Geometry check sheet. Reference: the model listing, model coordinates, mm. Face numbers are marked on the shaded views. A direction names the side the tool comes from. Give positions to 0.01 mm unless a question says otherwise; leave off trailing zeros. Loops run counter-clockwise (first coordinate to the right, second up) from the corner with the lowest first, then second, coordinate; pieces in that order, holes last. Notation, with made-up numbers: (81, 39) -> (104, 39) arc R15 ccw to (104, 68) -> close; hole circle Ø9 at (18.5, 88.5). An arc over 180 degrees is marked (long way). Write item = value, one per line.
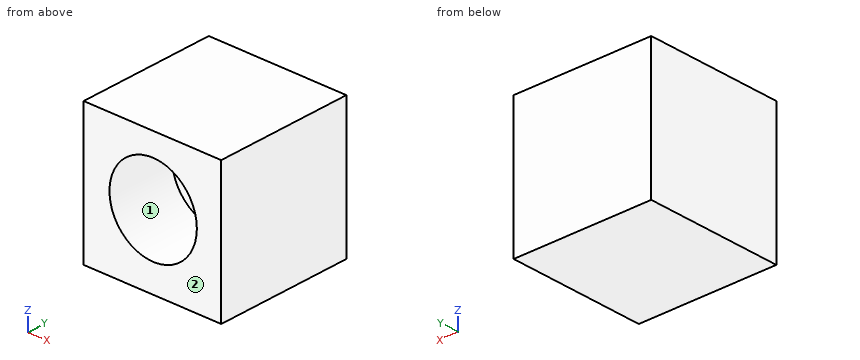
```python
from build123d import *

# Parameters (mm, degrees)
F0_W     = 76.2
F0_H     = 76.2
F1_DEPTH = 76.2
F2_R     = 24.198558
F3_DEPTH = 38.1


with BuildPart() as f1:
    # F0 (on Front) → F1 (new body)
    with BuildSketch(Plane.XZ):
        with Locations((-5.188912, 4.258561)):
            Rectangle(F0_W, F0_H)
    extrude(amount=F1_DEPTH)

    # F2 (on face) → F3 (cut, symmetric)
    with BuildSketch(Plane.XZ.offset(76.2)):
        with Locations((-4.792011, 5.650742)):
            Circle(F2_R)
    extrude(amount=F3_DEPTH, both=True, mode=Mode.SUBTRACT)


solid = f1.part
```
Item 1: Section check B-B, the plane z = 9.5. Record the cut outline in (x, y), plus the area to 3 significant figures.
Answer:
outline = (-43.29, -76.2) -> (-28.68, -76.2) -> (-28.68, -38.1) -> (19.1, -38.1) -> (19.1, -76.2) -> (32.91, -76.2) -> (32.91, 0) -> (-43.29, 0) -> close
area = 3,990 mm^2
Item 2: Tool access check on the marked faces 1 and 2. Record the directions out of +Z, -Z, +X, -X, +Y, -Y that give a thin tool (end or side, any length) a straight path to the whole face; none if there is none.
Answer:
face_1 = -Y
face_2 = +Z, -Z, +X, -X, -Y
Item 3: Section check A-A, the plane y = -52.5. Record the cut outline in (x, z), plus the area to 3 significant figures.
Answer:
outline = (-43.29, -33.84) -> (32.91, -33.84) -> (32.91, 42.36) -> (-43.29, 42.36) -> close; hole circle Ø48.4 at (-4.79, 5.65)
area = 3,970 mm^2
Item 4: Section check C-C, the plane x = -8.5. Record the cut outline in (y, z), plus the area to 3 significant figures.
Answer:
outline = (-76.2, -33.84) -> (0, -33.84) -> (0, 42.36) -> (-76.2, 42.36) -> (-76.2, 29.56) -> (-38.1, 29.56) -> (-38.1, -18.26) -> (-76.2, -18.26) -> close
area = 3,980 mm^2
Item 5: Thickness scan on L1, parallel to Y at x = -23, z = 5; L2, parallel to Z at x = 17.5, y = -71; L3, parallel to X at y = -72, z = 12. Record the ranges inside material, lowest first. Write a range as [from, to].
Answer:
L1 = [-38.1, 0]
L2 = [-33.84, -3.76], [15.07, 42.36]
L3 = [-43.29, -28.14], [18.56, 32.91]
